```python
from build123d import *

# Parameters (mm, degrees)
BOSS_EXTRUDE2_DEPTH      = 111.125
BOSS_EXTRUDE2_DEPTH_BACK = 111.125
SKETCH4_OUTSIDE_W        = 52.842
SKETCH4_OUTSIDE_H        = 53.824
SKETCH4_OUTSIDE_R        = 3.175
CUT_EXTRUDE1_DEPTH       = 15.24
SKETCH5_OUTSIDE_W        = 52.842
SKETCH5_OUTSIDE_H        = 53.824
SKETCH5_OUTSIDE_R        = 3.175
CUT_EXTRUDE4_DEPTH       = 15.24
SKETCH7_OUTSIDE_W        = 52.842
SKETCH7_OUTSIDE_H        = 53.824
SKETCH7_OUTSIDE_R        = 2.667
CUT_EXTRUDE8_DEPTH       = 0.762
SKETCH8_OUTSIDE_W        = 52.842
SKETCH8_OUTSIDE_H        = 53.824
SKETCH8_OUTSIDE_R        = 2.667
CUT_EXTRUDE9_DEPTH       = 0.762
BOSS_EXTRUDE4_DEPTH      = 11.43


with BuildPart() as part:
    # Sketch3 → Boss-Extrude2 (new, two sides: drawn at the far end of the back side and taken through both)
    with BuildSketch(Plane.XY.offset(-BOSS_EXTRUDE2_DEPTH_BACK)):
        Polygon((0, 3.666174209), (-3.175, 1.833087105), (-3.175, -1.833087105), (0, -3.666174209), (3.175, -1.833087105), (3.175, 1.833087105), align=None)
    extrude(amount=BOSS_EXTRUDE2_DEPTH + BOSS_EXTRUDE2_DEPTH_BACK)

    # Sketch4 outside → Cut-Extrude1 (cut)
    with BuildSketch(Plane.XY.offset(111.125)):
        Rectangle(SKETCH4_OUTSIDE_W, SKETCH4_OUTSIDE_H)
        Circle(SKETCH4_OUTSIDE_R, mode=Mode.SUBTRACT)
    extrude(amount=-CUT_EXTRUDE1_DEPTH, mode=Mode.SUBTRACT)

    # Sketch5 outside → Cut-Extrude4 (cut)
    with BuildSketch(Plane(origin=(0, 0, -111.125), x_dir=(-1, 0, 0), z_dir=(0, 0, -1))):
        Rectangle(SKETCH5_OUTSIDE_W, SKETCH5_OUTSIDE_H)
        with Locations(Location((0, 0, 0), (0, 0, 180))):
            Circle(SKETCH5_OUTSIDE_R, mode=Mode.SUBTRACT)
    extrude(amount=-CUT_EXTRUDE4_DEPTH, mode=Mode.SUBTRACT)

    # Sketch7 outside → Cut-Extrude8 (cut)
    with BuildSketch(Plane(origin=(0, 0, -107.823), x_dir=(-1, 0, 0), z_dir=(0, 0, -1))):
        Rectangle(SKETCH7_OUTSIDE_W, SKETCH7_OUTSIDE_H)
        with Locations(Location((0, 0, 0), (0, 0, 180))):
            Circle(SKETCH7_OUTSIDE_R, mode=Mode.SUBTRACT)
    extrude(amount=CUT_EXTRUDE8_DEPTH, mode=Mode.SUBTRACT)

    # Sketch8 outside → Cut-Extrude9 (cut)
    with BuildSketch(Plane.XY.offset(107.823)):
        Rectangle(SKETCH8_OUTSIDE_W, SKETCH8_OUTSIDE_H)
        Circle(SKETCH8_OUTSIDE_R, mode=Mode.SUBTRACT)
    extrude(amount=CUT_EXTRUDE9_DEPTH, mode=Mode.SUBTRACT)

    # Sketch13 → Boss-Extrude4 (add)
    with BuildSketch(Plane(origin=(0, 0, -111.125), x_dir=(-1, 0, 0), z_dir=(0, 0, -1))):
        Polygon((0, 3.666174278), (-3.175000059, 1.833087139), (-3.175000059, -1.833087139), (0, -3.666174278), (3.175000059, -1.833087139), (3.175000059, 1.833087139), align=None)
    extrude(amount=BOSS_EXTRUDE4_DEPTH)


solid = part.part
```
Verification items for the finished model (mm, model axes). A direction names the side the tool comes from. Give positions to 0.01 mm unless a question says otherwise; leave off trailing zeros. Order: outer loops, then holes, each group sorted by start corner. A loop starts at its lowest first (then second) coordinate and runs counter-clockwise, first axis right, second up. Notation, with made-up numbers: (-19.5, 71.25) -> (33.5, 71.25) arc R23 ccw to (33.5, 91.25) -> close; hole circle Ø2 at (65.5, 13.5). An arc over 180 degrees is marked (long way). One line per item, written item: value.
(1) Tool access check on faces 1 (the face through (1.231, -2.366, 108.199)), 2 (the face through (-3.175, 0, -1)), 3 (the face through (-0.69, -3.1, 101.94)). Record the directions out of +Z, -Z, +X, -X, +Y, -Y that give a thin tool (end or side, any length) a straight path to the whole face; none if there is none.
Final values:
face 1: none
face 2: +Z, -Z, -X, +Y, -Y
face 3: +Z
(2) Sectioned sample at A-A on z = -102.5. Record the cut outline in (x, y) (3 decimals).
Final values:
outline: circle Ø6.35 at (0, 0)
(3) Gauge pin test, flat ends, axial feed: pin 1 (0.8 mm diameter, centred on x = 2.5, y = -2, fed in from +Z) (3 decimals); pin 2 (0.5 mm diameter, centred on x = 0, y = 3.5, fed in from +Z) (3 decimals). Record the tip position at first contact, or that the pin passes through.
Final values:
pin 1: z = 111.125
pin 2: z = 95.885
(4) Scan lines: line 1 along Z through (x, y) = (1.5, 2.25) (3 decimals); line 2 along Z through (x, y) = (0, -3.25) (3 decimals); line 3 along Y through (x, z) = (-1.75, 50). Record each from-to range of solid material in increasing order. Write a range as [from, to].
Final values:
line 1: [-122.555, -108.585], [-107.823, 107.823], [108.585, 111.125]
line 2: [-122.555, -111.125], [-95.885, 95.885]
line 3: [-2.66, 2.66]
(5) Draft check along Z on faces 4 (the face through (0, 0, -122.555)), 5 (the face through (0, 0, 111.125)), 6 (the face through (-0.69, -3.1, 109.87)), 7 (the face through (2, 2, -107.823)). Enter one of: pulls with the +Z half, pulls with the -Z half, needs draft (parallel to the pull), parting line crosses it, or undercut.
Final values:
face 4: pulls with the -Z half
face 5: pulls with the +Z half
face 6: needs draft
face 7: undercut
